from build123d import *

# Parameters (mm, degrees)
F1_DEPTH = 25.4
F2_R     = 15.875
F3_R     = 4.826
F4_R     = 1.524


with BuildPart() as f1:
    # F0 (on Front) → F1 (new body)
    with BuildSketch(Plane.XZ):
        with BuildLine():
            Line((0, 4.7752), (0, 0))
            Line((0, 0), (67.9704, 0))
            Line((67.9704, 0), (67.9704, 4.7752))
            Line((67.9704, 4.7752), (67.9704, 27.0002))
            Line((67.9704, 27.0002), (74.3204, 27.0002))
            Line((74.3204, 27.0002), (74.3204, 31.7754))
            Line((74.3204, 31.7754), (67.9704, 31.7754))
            Line((67.9704, 31.7754), (63.1952, 31.7754))
            Line((63.1952, 31.7754), (63.1952, 14.3002))
            ThreePointArc((63.1952, 14.3002), (60.405392, 7.565008), (53.6702, 4.7752))
            Line((53.6702, 4.7752), (14.3002, 4.7752))
            ThreePointArc((14.3002, 4.7752), (7.565008, 7.565008), (4.7752, 14.3002))
            Line((4.7752, 14.3002), (4.7752, 31.7754))
            Line((4.7752, 31.7754), (0, 31.7754))
            Line((0, 31.7754), (-6.35, 31.7754))
            Line((-6.35, 31.7754), (-6.35, 27.0002))
            Line((-6.35, 27.0002), (0, 27.0002))
            Line((0, 27.0002), (0, 4.7752))
        make_face()
    extrude(amount=F1_DEPTH)

    # F2
    f2_edges = [f1.edges().sort_by_distance(p)[0] for p in [
        (0, -12.7, 0),
        (67.9704, -12.7, 0),
    ]]
    fillet(f2_edges, radius=F2_R)

    # F3
    f3_edges = [f1.edges().sort_by_distance(p)[0] for p in [
        (-6.35, 0, 29.3878),
        (-6.35, -25.4, 29.3878),
        (74.3204, 0, 29.3878),
        (74.3204, -25.4, 29.3878),
    ]]
    fillet(f3_edges, radius=F3_R)

    # F4
    f4_edges = [f1.edges().sort_by_distance(p)[0] for p in [
        (0, -12.7, 27.0002),
        (4.7752, -12.7, 31.7754),
        (63.1952, -12.7, 31.7754),
        (67.9704, -12.7, 27.0002),
    ]]
    fillet(f4_edges, radius=F4_R)


solid = f1.part
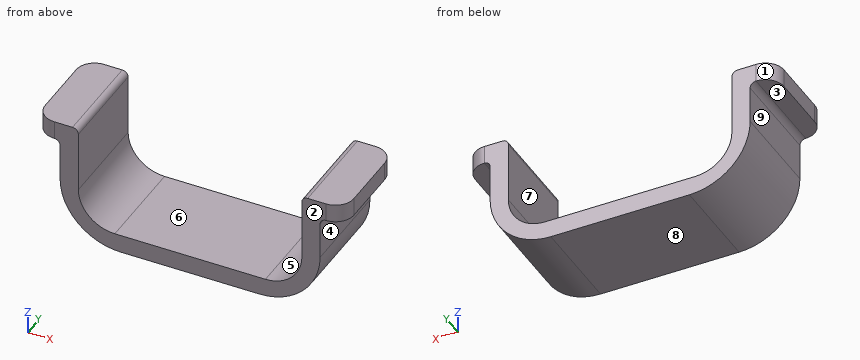
Verification items for the finished model (mm, model axes). Face numbers are marked on the shaded views. A direction names the side the tool comes from. Coordinates: 2 decimals unless noted, no trailing zeros. Loops run counter-clockwise (first coordinate to the right, second up) from the corner with the lowest first, then second, coordinate; pieces in that order, holes last. Notation, with made-up numbers: M 10.5,-9.75 L 64.5,-9.75 A15 ccw 64.5,-3.75 Z; hole C 79.25,43 d10. An arc over 180 degrees is marked long. One line per item, written item: value.
1. Section check D-D on z = 13.5. Record the cut outline in (x, y).
Answers follow:
outline: M 0.18,-25.4 L 4.81,-25.4 L 4.81,0 L 0.18,0 Z; M 63.16,-25.4 L 67.79,-25.4 L 67.79,0 L 63.16,0 Z
2. Gauge pin test, flat ends, axial feed: P1, Ø8, axis at y = -11, z = 21, coming from the +X side; P2, Ø4, axis at x = 38, y = -16, coming from the +Z side; P3, Ø2, axis at y = -9.5, z = 12.5, coming from the +X side; P4, Ø10, axis at x = 18.5, z = 14, coming from the +Y side. Record the tip position at first contact, or that the pin passes through.
Answers follow:
P1: x = 67.97
P2: z = 4.78
P3: x = 67.79
P4: through
3. Section check A-A on y = -9.75. Record the cut outline in (x, z) (3 decimals), plus the area to 3 significant figures.
Answers follow:
outline: M -6.35,27 L -1.524,27 A1.524 cw 0,25.476 L 0,15.875 A15.875 ccw 15.875,0 L 52.095,0 A15.875 ccw 67.97,15.875 L 67.97,25.476 A1.524 cw 69.494,27 L 74.32,27 L 74.32,31.775 L 64.719,31.775 A1.524 ccw 63.195,30.251 L 63.195,14.3 A9.525 cw 53.67,4.775 L 14.3,4.775 A9.525 cw 4.775,14.3 L 4.775,30.251 A1.524 ccw 3.251,31.775 L -6.35,31.775 Z
area: 574 mm^2
4. Set-up check for the marked faces 1, 2, 3, 4 and 5: record each of +Z, -Z, +X, -X, +Y, -Y from which the full face is reachable in a straight line by a thin tool's end or side.
Answers follow:
face 1: +Z, -Z, -X, +Y
face 2: +Z, -Z, +X, -X, -Y
face 3: -Z, -X, +Y, -Y
face 4: -Z, +X, +Y, -Y
face 5: +Z, +Y, -Y
5. Section check C-C on x = 36. Record the cut outline in (y, z), plus the area to 3 significant figures.
Answers follow:
outline: M -25.4,0 L 0,0 L 0,4.78 L -25.4,4.78 Z
area: 121 mm^2
6. Material ranges on line 1 along X through (y, z) = (-9.25, 21); line 2 along Z through (x, y) = (31, -15.5); line 3 along X through (y, z) = (-19, 29.5), recorded low to high. Write a range as from..to.
Answers follow:
line 1: 0..4.78, 63.2..67.97
line 2: 0..4.78
line 3: -6.35..4.78, 63.2..74.32
7. Mould release check, pull along X, two halves, no side actions. Record for the marked faces 6, 7, 8 and 9: pulls with the +X half, pulls with the -X half, needs draft (parallel to the pull), parting line crosses it, or undercut.
Answers follow:
face 6: undercut
face 7: undercut
face 8: needs draft
face 9: pulls with the -X half
8. Section check B-B on z = 8. Record the cut outline in (x, y).
Answers follow:
outline: M 2.09,-25.4 L 7.16,-25.4 L 7.16,0 L 2.09,0 Z; M 60.81,-25.4 L 65.88,-25.4 L 65.88,0 L 60.81,0 Z
